For this review, take the finished solid that the model builds, in its own axes (mm). A direction names the side the tool comes from. Give positions to 0.01 mm unless a question says otherwise; leave off trailing zeros. Order: outer loops, then holes, each group sorted by start corner. A loop starts at its lowest first (then second) coordinate and runs counter-clockwise, first axis right, second up.
from build123d import *

# Parameters (mm, degrees)
F3_R     = 9.7677281956
F3_R_2   = 7.6796646
F4_DEPTH = 86.2554833293
F5_DEPTH = 1.8415
F6_DEPTH = 5.08


# Not quite as in the source:
# - a fillet or chamfer that OpenCascade refuses, or shapes differently, is made with other operations: its cross-section is extruded or revolved along the edge and cut away or added


with BuildPart() as f1:
    # F0 (on Front) → F1 (revolve)
    with BuildSketch(Plane.XZ):
        with BuildLine():
            add(Edge.make_bspline(
                [(-16.0994362086, 126.6403571513), (-15.4416487906, 129.818912005), (-18.3602187314, 137.0481581434), (-30.7776463133, 151.6944538615), (-31.8157197837, 162.4649808678), (-32.0365097363, 167.6998246302)],
                knots=[0, 0, 0, 0, 0.2764092674, 0.6542388522, 1, 1, 1, 1], degree=3))
            Line((-16.0994362086, 126.6403571513), (-16.0994362086, 124.6616938849))
            Line((-16.0994362086, 124.6616938849), (-10.6212262798, 124.6616938849))
            Line((-10.6212262798, 124.6616938849), (-10.6212262798, 126.6403571513))
            Line((-10.6212262798, 126.6403571513), (-10.6212262798, 167.9538246302))
            Line((-10.6212262798, 167.9538246302), (-10.6212262798, 173.5984517965))
            Line((-10.6212262798, 173.5984517965), (-10.6212262798, 192.7077323198))
            Line((-10.6212262798, 192.7077323198), (-10.6212262798, 202.9486296068))
            Line((-10.6212262798, 202.9486296068), (-68.306534248, 202.9486296068))
            Line((-68.306534248, 202.9486296068), (-56.8935275078, 195.6928223372))
            Line((-56.8935275078, 195.6928223372), (-41.0592220724, 185.6261789799))
            add(Edge.make_bspline(
                [(-33.8192135096, 173.5984517965), (-33.9311976843, 175.7700643461), (-34.1712077818, 180.4243736831), (-38.663140823, 183.8166663782), (-41.0592220724, 185.6261789799)],
                knots=[0, 0, 0, 0, 0.4665812951, 1, 1, 1, 1], degree=3))
            Line((-33.8192135096, 173.5984517965), (-33.8192135096, 170.823040801))
            Line((-33.8192135096, 170.823040801), (-33.8192135096, 170.6639382431))
            Line((-33.8192135096, 170.6639382431), (-34.1753996909, 171.1073964834))
            Line((-34.1753996909, 171.1073964834), (-34.47479508, 171.1073964834))
            Line((-34.47479508, 171.1073964834), (-34.5564074814, 171.1073964834))
            Line((-34.5564074814, 171.1073964834), (-33.8073261082, 170.1312959194))
            Line((-33.8073261082, 170.1312959194), (-33.8073261082, 167.6998246302))
            Line((-33.8073261082, 167.6998246302), (-32.0365097363, 167.6998246302))
        make_face()
    revolve(axis=Axis((-2.9415616798, 0, 150.6240181996), (0, 0, 1)))

    # F2: fillet of radius 5.08 on 1 edges, made by hand

    # F2_s1 → F2_t2 (revolve)
    with BuildSketch(Plane.XZ):
        with BuildLine():
            ThreePointArc((-31.8196671786, 164.0759580259), (-32.4282830228, 166.0991776077), (-33.8073261082, 167.6998246302))
            Line((-33.8073261082, 167.6998246302), (-33.7458267391, 167.780697293))
            ThreePointArc((-33.7458267391, 167.780697293), (-32.9219179223, 167.8014246302), (-32.0365097363, 167.8014246302))
            Line((-32.0365097363, 167.8014246302), (-31.934999984, 167.704106006))
            ThreePointArc((-31.934999984, 167.704106006), (-31.8450405903, 165.8927492145), (-31.7184146309, 164.0843533567))
            Line((-31.7184146309, 164.0843533567), (-31.8196671786, 164.0759580259))
        make_face()
    revolve(axis=Axis((-2.9415616798, 0, 167.6998246302), (0, 0, 1)))

    # F3 (on face) → F4 (cut)
    with BuildSketch(Plane.XY.offset(202.9486296068)):
        with Locations((-2.9415616798, 0)):
            Circle(F3_R)
        with Locations((-2.9415616798, 0)):
            Circle(F3_R_2, mode=Mode.SUBTRACT)
    extrude(amount=-F4_DEPTH, mode=Mode.SUBTRACT)

    # F3 (on face) → F5 (cut)
    with BuildSketch(Plane.XY.offset(202.9486296068)):
        with BuildLine():
            Line((-37.0871919824, 14.1988984612), (33.7026080176, 14.1988984612))
            Line((33.7026080176, 14.1988984612), (33.7026080176, 54.127483463))
            ThreePointArc((33.7026080176, 54.127483463), (-1.4554201029, 65.3480758864), (-37.0871919824, 55.7373803661))
            Line((-37.0871919824, 55.7373803661), (-37.0871919824, 14.1988984612))
        make_face()
    extrude(amount=-F5_DEPTH, mode=Mode.SUBTRACT)

    # F3 (on face) → F6 (cut)
    with BuildSketch(Plane.XY.offset(202.9486296068)):
        with BuildLine():
            Line((-42.164, -12.5023329654), (-42.164, -52.2893867918))
            ThreePointArc((-42.164, -52.2893867918), (0.9127584674, -65.2512364254), (42.164, -47.3082227989))
            Line((42.164, -47.3082227989), (42.164, -12.5023329654))
            Line((42.164, -12.5023329654), (-42.164, -12.5023329654))
        make_face()
    extrude(amount=-F6_DEPTH, mode=Mode.SUBTRACT)


solid = f1.part
1) Draft analysis for pull direction X (two halves, no side actions). For faces 5 (the face through (-32.382, -9.271, 168.899)), 6 (the face through (-42.164, -28, 200)), 7 (the face through (-4, 13, 202.949)), 8 (the face through (-5.059, -9.535, 164.353)), state which applies: +X half, -X half, draft (parallel to the pull), parting line (faces both ways), or undercut.
Answer sheet:
face 5: parting line
face 6: undercut
face 7: draft
face 8: undercut
2) Clearance check with flat-ended pins moving along their axes: pin 1 (5.5 mm diameter, centred on y = -23.5, z = 201, fed in from +X); pin 2 (0.9 mm diameter, centred on y = 41.5, z = 202.5, fed in from +X); pin 3 (2 mm diameter, centred on y = 11, z = 157, fed in from -X). State where each tip first meets the part, or that it passes through.
Answer sheet:
pin 1: stops at x = 58.77
pin 2: stops at x = 47.63
pin 3: stops at x = -28.91
3) To check wall thickness, follow line 1 (Y direction, x = 21.5, z = 171); line 2 (X direction, y = -1, z = 185); line 3 (Y direction, x = -7, z = 135). State the ranges of each line that lie inside material, in increasing order.
Answer sheet:
line 1: y = -19.92 to -19.31, -18.87 to 18.87, 19.31 to 19.92
line 2: x = -40.22 to -12.66, 6.77 to 34.34
line 3: y = -14.54 to -8.88, 8.88 to 14.54
4) Tool access review of faces 1 (the face through (-1, -35, 197.869)), 2 (the face through (7.5, 8.006, 125.637)), 3 (the face through (-2, 39, 201.107)), 4 (the face through (-33.5, -7.2, 171.107)): name each direction out of +Z, -Z, +X, -X, +Y, -Y from which nothing blocks a thin tool from reaching the whole face with its end or side.
Answer sheet:
face 1: +Z, -Y
face 2: -Z
face 3: +Z, +Y
face 4: none
5) We need section A-A on z = 188.5. Give the boundary of the cut face in (x, y).
Answer sheet:
outline: circle Ø85.28 at (-2.94, 0); hole circle Ø19.54 at (-2.94, 0)
